from build123d import *

# Parameters (mm, degrees)
SKETCH1_R           = 1.5
SKETCH1_W           = 12
SKETCH1_H           = 4.5
SKETCH1_H_2         = 3.5
BOSS_EXTRUDE1_DEPTH = 6
SKETCH3_W           = 3
SKETCH3_H           = 35
BOSS_EXTRUDE2_DEPTH = 2


with BuildPart() as part:
    # Sketch1 → Boss-Extrude1 (new body)
    # profile 1 of 4: a face of its own
    with BuildSketch(Plane(origin=(0, 0, 0), x_dir=(1, 0, 0), z_dir=(0, 1, 0))):
        with BuildLine():
            Line((11, -4), (-11, -4))
            ThreePointArc((-11, -4), (-15, 0), (-11, 4))
            Line((-11, 4), (11, 4))
            ThreePointArc((11, 4), (15, 0), (11, -4))
        make_face()
        with Locations(Location((11, 0, 0), (0, 0, 270))):
            Circle(SKETCH1_R, mode=Mode.SUBTRACT)
        with Locations(Location((-11, 0, 0), (0, 0, 270))):
            Circle(SKETCH1_R, mode=Mode.SUBTRACT)
    # profile 2 of 4: a face of its own
    with BuildSketch(Plane(origin=(0, 0, 0), x_dir=(1, 0, 0), z_dir=(0, 1, 0))):
        with Locations((0, 6.25)):
            Rectangle(SKETCH1_W, SKETCH1_H)
    # profile 3 of 4: a face of its own
    with BuildSketch(Plane(origin=(0, 0, 0), x_dir=(1, 0, 0), z_dir=(0, 1, 0))):
        with Locations((0, -5.75)):
            Rectangle(SKETCH1_W, SKETCH1_H_2)
    # profile 4 of 4: a face of its own
    with BuildSketch(Plane(origin=(0, 0, 0), x_dir=(1, 0, 0), z_dir=(0, 1, 0))):
        with BuildLine():
            Line((6, -47), (6, -51.5))
            Line((6, -51.5), (-6, -51.5))
            Line((-6, -51.5), (-6, -47))
            Line((-6, -47), (-11, -47))
            ThreePointArc((-11, -47), (-15, -43), (-11, -39))
            Line((-11, -39), (-6, -39))
            Line((-6, -39), (-6, -35.5))
            Line((-6, -35.5), (6, -35.5))
            Line((6, -35.5), (6, -39))
            Line((6, -39), (11, -39))
            ThreePointArc((11, -39), (15, -43), (11, -47))
            Line((11, -47), (6, -47))
        make_face()
        with Locations(Location((-11, -43, 0), (0, 0, 90))):
            Circle(SKETCH1_R, mode=Mode.SUBTRACT)
        with Locations(Location((11, -43, 0), (0, 0, 90))):
            Circle(SKETCH1_R, mode=Mode.SUBTRACT)
    extrude(amount=BOSS_EXTRUDE1_DEPTH)

    # Sketch3 → Boss-Extrude2 (add)
    with BuildSketch(Plane(origin=(0, 6, 0), x_dir=(1, 0, 0), z_dir=(0, 1, 0))):
        with Locations((7.5, -21.5)):
            Rectangle(SKETCH3_W, SKETCH3_H)
        with Locations((-7.5, -21.5)):
            Rectangle(SKETCH3_W, SKETCH3_H)
    extrude(amount=-BOSS_EXTRUDE2_DEPTH)


solid = part.part
Can you work these out from the model? Positions are in its coordinate system, mm. A direction names the side the tool comes from. Coordinates: 2 decimals unless noted, no trailing zeros. Write each loop counter-clockwise with the first axis right and the second up, starting at its lowest first coordinate (ties: lowest second). Pieces come first, ordered by that corner, then holes. Notation, with made-up numbers: (57.25, 80.25) -> (92.25, 80.25) arc R16 cw to (92.25, 108.25) -> close; hole circle Ø5 at (5.5, 51.5). An arc over 180 degrees is marked (long way). Answer as CSV lines item,"result".
1) If we section it at C-C on z = 43: Please give me the cut outline in (x, y).
Check result:
outline,"(-15, 0) -> (-12.5, 0) -> (-12.5, 6) -> (-15, 6) -> close; (-9.5, 0) -> (9.5, 0) -> (9.5, 6) -> (-9.5, 6) -> close; (12.5, 0) -> (15, 0) -> (15, 6) -> (12.5, 6) -> close"
2) If I drill on line 1 (X direction, y = 3.45, z = 0); line 2 (X direction, y = 2.1, z = 44); line 3 (Z direction, x = 8.5, y = 1.35), over which ranges is the centre line in solid material (lowest first)? Write a range as from..to.
Check result:
line 1,"-15..-12.5, -9.5..9.5, 12.5..15"
line 2,"-14.87..-12.12, -9.88..9.88, 12.12..14.87"
line 3,"-4..4, 39..47"
3) If we mould it in two halves opening along Z, with no side actions, what happens to faces 6 (the flat face through (-9, 3, -4)), 7 (the cylindrical face through (15, 3, 43)), 8 (the flat face through (0, 0, -1)), 9 (the flat face through (9, 3, 47))? For each: +Z half, -Z half, draft (parallel to the pull), parting line (faces both ways), or undercut.
Check result:
face 6,"-Z half"
face 7,"undercut"
face 8,"draft"
face 9,"+Z half"
4) On a 3-axis mill with a long thin cutter (end or side, diameter ignored), from which of +Z, -Z, +X, -X, +Y, -Y can I reach the whole of each face in a straight line? I mean faces 1 (the flat face through (9, 5, 22)), 2 (the flat face through (-6, 3, -6)), 3 (the flat face through (-6, 2, 37)), 4 (the flat face through (8, 2, 39)), 5 (the flat face through (6, 3, 49)). Say none if no direction works.
Check result:
face 1,"+X, +Y, -Y"
face 2,"-Z, -X, +Y, -Y"
face 3,"-X, -Y"
face 4,"+X, -Y"
face 5,"+Z, +X, +Y, -Y"
5) If we section it at A-A on x = -1.75: Please give me the cut outline in (y, z), then the cut area to 3 significant figures.
Check result:
outline,"(0, -8.5) -> (6, -8.5) -> (6, 7.5) -> (0, 7.5) -> close; (0, 35.5) -> (6, 35.5) -> (6, 51.5) -> (0, 51.5) -> close"
area,"192 mm²"
6) Will these pins go through, and if not, where does the flat tip stop? P1, Ø2, axis at y = 2, z = -6.5, coming from the -X side; P2, Ø3, axis at y = 2.5, z = 5, coming from the -X side; P3, Ø0.6, axis at y = 5, z = 22.5, coming from the +X side; P4, Ø3.5, axis at x = 11, z = 43, coming from the +Y side.
Check result:
P1,"x = -6"
P2,"x = -12.94"
P3,"x = 9"
P4,"y = 6"
7) If we section it at D-D on z = 28.5: Please give me the cut outline in (x, y).
Check result:
outline,"(-9, 4) -> (-6, 4) -> (-6, 6) -> (-9, 6) -> close; (6, 4) -> (9, 4) -> (9, 6) -> (6, 6) -> close"
8) If we section it at B-B on y = 0.55: Please give me the cut outline in (x, z), then the cut area to 3 significant figures.
Check result:
outline,"(-11, -4) -> (-6, -4) -> (-6, -8.5) -> (6, -8.5) -> (6, -4) -> (11, -4) arc R4 ccw to (11, 4) -> (6, 4) -> (6, 7.5) -> (-6, 7.5) -> (-6, 4) -> (-11, 4) arc R4 ccw to start; (-11, 39) -> (-6, 39) -> (-6, 35.5) -> (6, 35.5) -> (6, 39) -> (11, 39) arc R4 ccw to (11, 47) -> (6, 47) -> (6, 51.5) -> (-6, 51.5) -> (-6, 47) -> (-11, 47) arc R4 ccw to start; hole circle Ø3 at (-11, 0); hole circle Ø3 at (-11, 43); hole circle Ø3 at (11, 0); hole circle Ø3 at (11, 43)"
area,"616 mm²"
